The listing builds one solid part. Answer for the finished solid, in the listing's coordinates (mm). Face numbers are marked on the shaded views. A direction names the side the tool comes from. Coordinates: 2 decimals unless noted, no trailing zeros. Write each loop counter-clockwise with the first axis right and the second up, starting at its lowest first coordinate (ties: lowest second). Pieces come first, ordered by that corner, then holes.
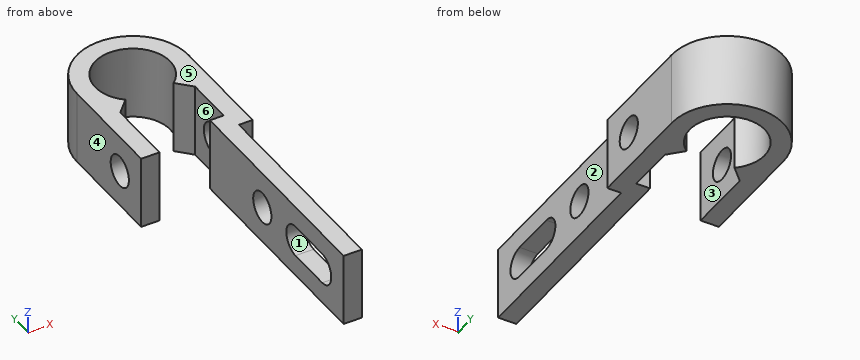
from build123d import *

# Parameters (mm, degrees)
RESSALTO_EXTRUS_O1_DEPTH = 8
ESBO_O2_R                = 1.7
CORTE_EXTRUS_O1_DEPTH    = 38.918860742


with BuildPart() as part:
    # Esboço1 → Ressalto-extrusão1 (new body)
    with BuildSketch(Plane.XY):
        with BuildLine():
            Line((4.1, -4.676945082), (2.6354292, -3.140782217))
            ThreePointArc((2.6354292, -3.140782217), (0, 4.1), (-2.6354292, -3.140782217))
            Line((-2.6354292, -3.140782217), (-4.1, -4.676945082))
            Line((-4.1, -4.676945082), (-4.1, -12))
            Line((-4.1, -12), (-6.1, -12))
            Line((-6.1, -12), (-6.1, 0))
            ThreePointArc((-6.1, 0), (0, 6.1), (6.1, 0))
            Line((6.1, 0), (6.1, -12))
            Line((6.1, -12), (4.6, -12))
            Line((4.6, -12), (4.6, -35))
            Line((4.6, -35), (2.6, -35))
            Line((2.6, -35), (2.6, -10))
            Line((2.6, -10), (4.1, -10))
            Line((4.1, -10), (4.1, -4.676945082))
        make_face()
    extrude(amount=RESSALTO_EXTRUS_O1_DEPTH)

    # Esboço2 → Corte-extrusão1 (cut, through all)
    with BuildSketch(Plane.ZY.offset(6.1)):
        with Locations((4, -8)):
            Circle(ESBO_O2_R)
        with Locations(Location((4, -19.8, 0), (0, 0, 270))):
            Circle(ESBO_O2_R)
        with BuildLine():
            Line((5.7, -26), (5.7, -31))
            ThreePointArc((5.7, -31), (4, -32.7), (2.3, -31))
            Line((2.3, -31), (2.3, -26))
            ThreePointArc((2.3, -26), (4, -24.3), (5.7, -26))
        make_face()
    extrude(amount=-CORTE_EXTRUS_O1_DEPTH, mode=Mode.SUBTRACT)


solid = part.part
1. Section C-C on z = 4.75 is taken. State how many separate pieces and enclosed holes the cut face has, then the cut area to 3 significant figures.
Results found:
separate pieces: 5
enclosed holes: 0
area: 99.7 mm2
2. Section D-D on y = -1.5 is taken. Give the vertices of the cut face in (x, z), then the cut area to 3 significant figures.
Results found:
outline: (-6.1, 0) - (-3.82, 0) - (-3.82, 8) - (-6.1, 8) - close; (3.82, 0) - (6.1, 0) - (6.1, 8) - (3.82, 8) - close
area: 36.5 mm2
3. Section B-B on y = -21 is taken. Give the vertices of the cut face in (x, z), then the cut area to 3 significant figures.
Results found:
outline: (2.6, 0) - (4.6, 0) - (4.6, 2.8) - (2.6, 2.8) - close; (2.6, 5.2) - (4.6, 5.2) - (4.6, 8) - (2.6, 8) - close
area: 11.2 mm2
4. A tool of negligible diameter and unlimited length cuts with its end or side. For the marked faces 1, 2 and 3, from which of +Z, -Z, +X, -X, +Y, -Y can it reach the whole face along a straight path? Write none if from no direction.
Results found:
face 1: +X, -X
face 2: +Z, -Z, +X, -Y
face 3: +Z, -Z, -Y
5. Flat-ended cylindrical pins translate along their axes: P1, Ø0.8, axis at x = 5.5, z = 3, coming from the -Y side; P2, Ø2, axis at x = 1.5, z = 7, coming from the -Y side; P3, Ø2.5, axis at y = -8, z = 4, coming from the -X side; P4, Ø1, axis at x = -3.5, z = 4.5, coming from the -Y side. Find the tip coordinate at first contact, or state that the pin passes through.
Results found:
P1: stops at y = -12
P2: stops at y = 3.25
P3: passes through
P4: stops at y = -4.57
6. Find the intervals of material crossed by L1, parallel to Z at x = 4, y = -19.8; L2, parallel to X at y = 0, z = 3; L3, parallel to X at y = -19, z = 7, in increasing order.
Results found:
L1: z = 0 to 2.3, 5.7 to 8
L2: x = -6.1 to -4.1, 4.1 to 6.1
L3: x = 2.6 to 4.6
7. Section A-A on y = -8 is taken. Give the vertices of the cut face in (x, z).
Results found:
outline: (-6.1, 0) - (-4.1, 0) - (-4.1, 2.3) - (-6.1, 2.3) - close; (-6.1, 5.7) - (-4.1, 5.7) - (-4.1, 8) - (-6.1, 8) - close; (4.1, 0) - (6.1, 0) - (6.1, 2.3) - (4.1, 2.3) - close; (4.1, 5.7) - (6.1, 5.7) - (6.1, 8) - (4.1, 8) - close
8. For a pull along X with two mould halves and no side action, classify the marked faces 4, 5 and 6 as pulls with the +X half, pulls with the -X half, needs draft (parallel to the pull), parting line crosses it, or undercut.
Results found:
face 4: pulls with the -X half
face 5: needs draft
face 6: undercut
